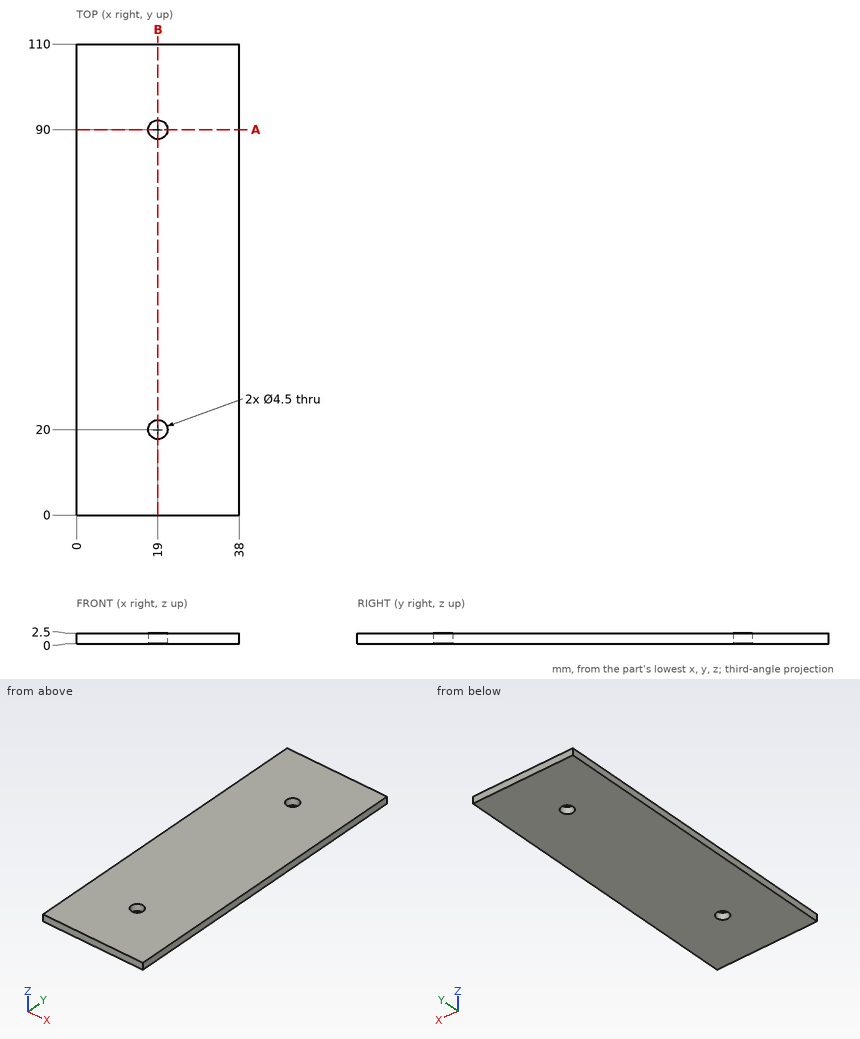
Could you check a few things on this drawing? It's one solid part, dimensions in mm from its lowest x, y, z. Round coordinates to 2 decimals unless told otherwise and drop trailing zeros. Write each loop counter-clockwise with the first axis right and the second up, starting at its lowest first coordinate (ties: lowest second). Pieces come first, ordered by that corner, then holes.
Q1. Please list where these lines run through material, in increasing order: probe 1 along Y at (x, z) = (19, 2); probe 2 along X at (y, z) = (20, 1.45).
Q2. If we section it at B-B on x = 19: Write out the boundary of the cut face in (y, z), plus the area to 4 significant figures.
Q3. Will these pins go through, and if not, where does the flat tip stop? P1, Ø5, axis at x = 19, y = 20, coming from the +Z side; P2, Ø2.5, axis at x = 19, y = 90, coming from the +Z side.
Q4. If we section it at A-A on y = 90: Write out the boundary of the cut face in (x, z), plus the area to 4 significant figures.
Answer below:
1. probe 1: y = 0 to 17.75, 22.25 to 87.75, 92.25 to 110
1. probe 2: x = 0 to 16.75, 21.25 to 38
2. outline: (0, 0) - (17.75, 0) - (17.75, 2.5) - (0, 2.5) - close; (22.25, 0) - (87.75, 0) - (87.75, 2.5) - (22.25, 2.5) - close; (92.25, 0) - (110, 0) - (110, 2.5) - (92.25, 2.5) - close
2. area: 252.5 mm2
3. P1: stops at z = 2.5
3. P2: passes through
4. outline: (0, 0) - (16.75, 0) - (16.75, 2.5) - (0, 2.5) - close; (21.25, 0) - (38, 0) - (38, 2.5) - (21.25, 2.5) - close
4. area: 83.75 mm2
